The model under review builds one solid part; all positions refer to its coordinate system, in mm. A direction names the side the tool comes from. Coordinates: 2 decimals unless noted, no trailing zeros. Loops run counter-clockwise (first coordinate to the right, second up) from the corner with the lowest first, then second, coordinate; pieces in that order, holes last. Notation, with made-up numbers: M 39.25,-13 L 50.25,-13 A20 ccw 50.25,-6 Z; hole C 3,39.5 d11. An arc over 180 degrees is marked long. Use CSV: the item, a comma, the result in double quotes. Start each with the question number.
from build123d import *

# Parameters (mm, degrees)
BOSS_EXTRUDE1_DEPTH = 10
FILLET1_R           = 3
SKETCH2_W           = 18
SKETCH2_H           = 10
BOSS_EXTRUDE2_DEPTH = 120


with BuildPart() as part:
    # Sketch1 → Boss-Extrude1 (new body)
    with BuildSketch(Plane.XY):
        Polygon((-9, 0), (9, 0), (9, 20), (3.99, 20), (3.99, 31), (9, 31), (9, 40), (3.99, 40), (3.99, 51), (9, 51), (9, 60), (3.99, 60), (3.99, 71), (9, 71), (9, 80), (3.99, 80), (3.99, 91), (9, 91), (9, 100), (3.99, 100), (3.99, 111), (9, 111), (9, 120), (3.99, 120), (-3.99, 120), (-9, 120), (-9, 111), (-3.99, 111), (-3.99, 100), (-9, 100), (-9, 91), (-3.99, 91), (-3.99, 80), (-9, 80), (-9, 71), (-3.99, 71), (-3.99, 60), (-9, 60), (-9, 51), (-3.99, 51), (-3.99, 40), (-9, 40), (-9, 31), (-3.99, 31), (-3.99, 20), (-9, 20), align=None)
    extrude(amount=BOSS_EXTRUDE1_DEPTH)

    # Fillet1
    fillet1_edges = [part.edges().sort_by_distance(p)[0] for p in [
        (-9, 31, 5),
        (-9, 40, 5),
        (-9, 51, 5),
        (-9, 60, 5),
        (-9, 71, 5),
        (-9, 80, 5),
        (-9, 91, 5),
        (-9, 100, 5),
        (-9, 111, 5),
        (9, 111, 5),
        (9, 100, 5),
        (9, 91, 5),
        (9, 80, 5),
        (9, 71, 5),
        (9, 60, 5),
        (9, 51, 5),
        (9, 40, 5),
        (9, 31, 5),
        (9, 0, 5),
        (-9, 0, 5),
    ]]
    fillet(fillet1_edges, radius=FILLET1_R)

    # Sketch2 → Boss-Extrude2 (add)
    with BuildSketch(Plane(origin=(0, 120, 0), x_dir=(1, 0, 0), z_dir=(0, 1, 0))):
        with Locations((0, -5)):
            Rectangle(SKETCH2_W, SKETCH2_H)
    extrude(amount=BOSS_EXTRUDE2_DEPTH)


solid = part.part
1. Insertion check: pin 1 Ø5 at (y, z) = (107, 6.5) entering from +X; pin 2 Ø3 at (y, z) = (63.5, 5.5) entering from -X; pin 3 Ø8 at (x, y) = (-4, 31) entering from -Z. Each pin has a flat end and moves straight along its axis. Give the tip position at first contact, or say it passes through.
2. To check wall thickness, follow line 1 along Y through (x, z) = (-5, 6.25); line 2 along Y through (x, z) = (-8, 6); line 3 along X through (y, z) = (88.5, 4.5). State the ranges of each line that lie inside material, in increasing order.
3. Add section A-A (y = 67). Write out the cut boundary in (x, z), plus the area to 3 significant figures.
4. Draft analysis for pull direction Y (two halves, no side actions). For faces 1 (the flat face through (0, 240, 5)), 2 (the flat face through (3.99, 45, 5)), 3 (the flat face through (-9, 176, 5)), 4 (the flat face through (0, 0, 5)), state which applies: released by +Y, released by -Y, zero draft, split by the parting line, or undercut.
5. For faces 5 (the flat face through (7, 20, 5)), 6 (the flat face through (9, 11, 5)), 7 (the flat face through (-3.99, 26, 5)), list the 3-axis set-ups (+Z, -Z, +X, -X, +Y, -Y) from which the entire face can be reached by the end or side of a thin tool; tool diameter is ignored.
Solved:
1,pin 1,"stops at x = 3.99"
1,pin 2,"stops at x = -3.99"
1,pin 3,"stops at z = 0"
2,line 1,"y = 0 to 20, 31 to 40, 51 to 60, 71 to 80, 91 to 100, 111 to 240"
2,line 2,"y = 0.76 to 20, 31.76 to 39.24, 51.76 to 59.24, 71.76 to 79.24, 91.76 to 99.24, 111.76 to 240"
2,line 3,"x = -3.99 to 3.99"
3,outline,"M -3.99,0 L 3.99,0 L 3.99,10 L -3.99,10 Z"
3,area,"79.8 mm^2"
4,face 1,"released by +Y"
4,face 2,"undercut"
4,face 3,"zero draft"
4,face 4,"released by -Y"
5,face 5,"+Z, -Z, +X"
5,face 6,"+Z, -Z, +X, +Y, -Y"
5,face 7,"+Z, -Z, -X"
